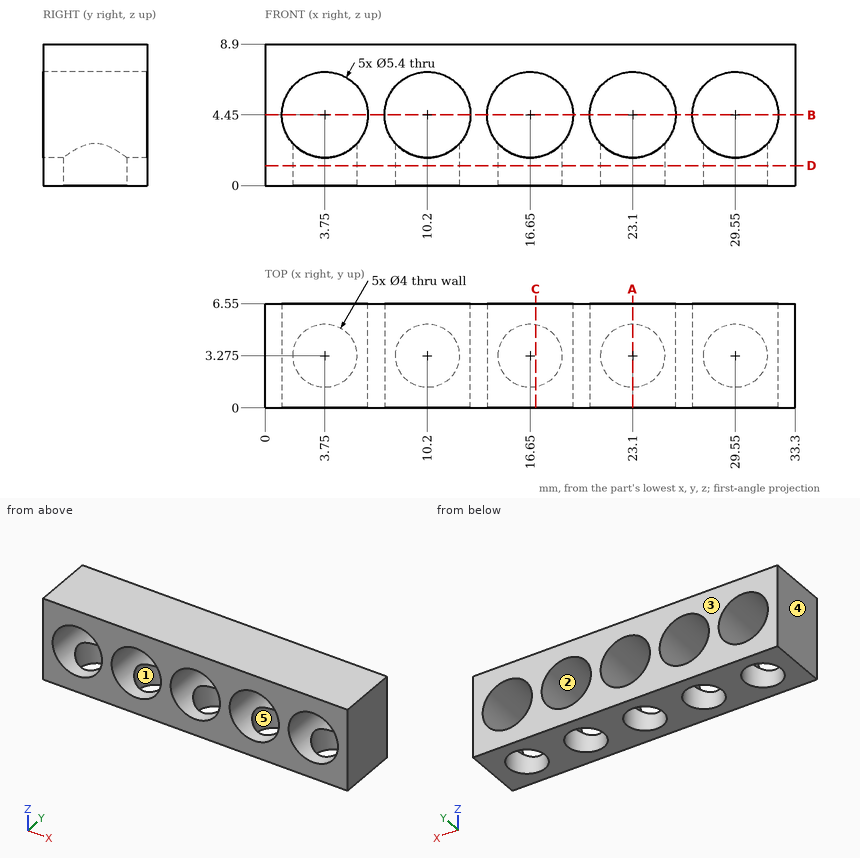
Can you work these out from the drawing? Everything is in mm from the part's minimum corner. A direction names the side the tool comes from. Round coordinates to 2 decimals unless told otherwise and drop trailing zeros. Write each loop counter-clockwise with the first axis right and the second up, starting at its lowest first coordinate (ties: lowest second). Pieces come first, ordered by that corner, then holes. Notation, with made-up numbers: M 88,-19 L 110,-19 A9 cw 110,-12 Z; hole C 68,39 d9. An arc over 180 degrees is marked long. Use a Markdown table: item, result.
Item 1: We'd pull the mould along X, two halves only. Please class the marked faces 3, 4 and 5: released by +X, released by -X, zero draft, split by the parting line, or undercut.
Found:
| item | result |
|---|---|
| face 3 | zero draft |
| face 4 | released by -X |
| face 5 | undercut |
Item 2: I want a section at B-B (z = 4.45). List the corners of the cut face in (x, y) for me.
Found:
| item | result |
|---|---|
| outline | M 0,0 L 1.05,0 L 1.05,6.55 L 0,6.55 Z; M 6.45,0 L 7.5,0 L 7.5,6.55 L 6.45,6.55 Z; M 12.9,0 L 13.95,0 L 13.95,6.55 L 12.9,6.55 Z; M 19.35,0 L 20.4,0 L 20.4,6.55 L 19.35,6.55 Z; M 25.8,0 L 26.85,0 L 26.85,6.55 L 25.8,6.55 Z; M 32.25,0 L 33.3,0 L 33.3,6.55 L 32.25,6.55 Z |
Item 3: Which directions (+Z, -Z, +X, -X, +Y, -Y) give clear straight access to the entire face, cutting with the end or side of a thin tool? Please do the marked faces 1 and 2.
Found:
| item | result |
|---|---|
| face 1 | -Z |
| face 2 | +Y, -Y |
Item 4: For pin 1 Ø5 at (x, z) = (29.55, 4.45) entering from +Y (1 decimal); pin 2 Ø2 at (y, z) = (3, 8) entering from -X; pin 3 Ø2.5 at (x, y) = (3.75, 3.275) entering from -Z, each with a flat end and sliding along its axis, tell me the tip position at first contact or that it passes through.
Found:
| item | result |
|---|---|
| pin 1 | passes through |
| pin 2 | stops at x = 0 |
| pin 3 | stops at z = 6.84 |
Item 5: I want a section at A-A (x = 23.1). List the corners of the cut face in (y, z) for me (3 decimals), and give its area (3 significant figures).
Found:
| item | result |
|---|---|
| outline | M 0,0 L 1.275,0 L 1.275,1.75 L 0,1.75 Z; M 0,7.15 L 6.55,7.15 L 6.55,8.9 L 0,8.9 Z; M 5.275,0 L 6.55,0 L 6.55,1.75 L 5.275,1.75 Z |
| area | 15.9 mm2 |
Item 6: If I drill on line 1 along X through (y, z) = (5.5, 4.25); line 2 along Y through (x, z) = (10.2, 0.9) (3 decimals); line 3 along X through (y, z) = (1.75, 6.25), over which ranges is the centre line in solid material (lowest first)? Write a range as [from, to].
Found:
| item | result |
|---|---|
| line 1 | x = [0, 1.06], [6.44, 7.51], [12.89, 13.96], [19.34, 20.41], [25.79, 26.86], [32.24, 33.3] |
| line 2 | y = [0, 1.275], [5.275, 6.55] |
| line 3 | x = [0, 1.74], [5.76, 8.19], [12.21, 14.64], [18.66, 21.09], [25.11, 27.54], [31.56, 33.3] |
Item 7: I want a section at C-C (x = 17). List the corners of the cut face in (y, z) for me, and give its area (3 significant figures).
Found:
| item | result |
|---|---|
| outline | M 0,0 L 1.31,0 L 1.31,1.77 L 0,1.77 Z; M 0,7.13 L 6.55,7.13 L 6.55,8.9 L 0,8.9 Z; M 5.24,0 L 6.55,0 L 6.55,1.77 L 5.24,1.77 Z |
| area | 16.2 mm2 |
Item 8: I want a section at D-D (z = 1.25). List the corners of the cut face in (x, y) for me (3 decimals).
Found:
| item | result |
|---|---|
| outline | M 0,0 L 33.3,0 L 33.3,6.55 L 0,6.55 Z; hole C 3.75,3.275 d4; hole C 10.2,3.275 d4; hole C 16.65,3.275 d4; hole C 23.1,3.275 d4; hole C 29.55,3.275 d4 |
